```python
from build123d import *

# Parameters (mm, degrees)
F0_R     = 53.6575
F1_DEPTH = 127
F2_R     = 48.26
F3_DEPTH = 118.11
F4_R     = 5.08
F5_R     = 5.08


with BuildPart() as f1:
    # F0 (on Top) → F1 (new body)
    with BuildSketch(Plane.XY):
        Circle(F0_R)
    extrude(amount=F1_DEPTH)

    # F2 (on face) → F3 (cut)
    with BuildSketch(Plane.XY.offset(127)):
        Circle(F2_R)
    extrude(amount=-F3_DEPTH, mode=Mode.SUBTRACT)

    # F4
    f4_edges = [f1.edges().sort_by_distance(p)[0] for p in [
        (-53.6575, 0, 127),
    ]]
    fillet(f4_edges, radius=F4_R)

    # F5
    f5_edges = [f1.edges().sort_by_distance(p)[0] for p in [
        (-53.6575, 0, 0),
    ]]
    fillet(f5_edges, radius=F5_R)


solid = f1.part
```
The listing builds one solid part. Answer for the finished solid, in the listing's coordinates (mm). Give positions to 0.01 mm unless a question says otherwise; leave off trailing zeros. Order: outer loops, then holes, each group sorted by start corner. A loop starts at its lowest first (then second) coordinate and runs counter-clockwise, first axis right, second up. Notation, with made-up numbers: (-38, -35) - (1, -35) arc R20 cw to (1, -14) - close; hole circle Ø2 at (70.25, 46.5). An arc over 180 degrees is marked (long way). Answer in a Markdown table with one row per item. Add a question column.
Q1. Given P1, Ø1, axis at x = -1, y = 29.5, coming from the +Z side; P2, Ø12, axis at x = -38.5, y = 40.5, coming from the -Z side; P3, Ø1.5, axis at x = -13.5, z = 92.5, coming from the -Y side, each flat-ended and moving along its own axis, determine where each tip first touches the part or whether it passes through.
Q2. For a pull along Z with two mould halves and no side action, classify faces 1 (the flat face through (-1, 1, 8.89)), 2 (the flat face through (-1, 1, 0)), 3 (the cylindrical face through (46.03, 14.5, 68.77)) as released by +Z, released by -Z, zero draft, split by the parting line, or undercut.
Q3. Find the intervals of material crossed by line 1 along Y through (x, z) = (0, 77.5); line 2 along Z through (x, y) = (-3, 45); line 3 along X through (y, z) = (42.5, 77.5), in increasing order. Write a range as [from, to].
Q4. The part is cut by section C-C (z = 16.5). Determine the outline of the cut face in (x, y) (1 decimal), then the cut area to 3 significant figures.
Q5. The part is cut by section A-A (x = 0). Determine the outline of the cut face in (y, z), then the cut area to 3 significant figures.
Determined:
| question | item | result |
|---|---|---|
| 1 | P1 | stops at z = 8.89 |
| 1 | P2 | stops at z = 0.17 |
| 1 | P3 | stops at y = -52.12 |
| 2 | face 1 | released by +Z |
| 2 | face 2 | released by -Z |
| 2 | face 3 | zero draft |
| 3 | line 1 | y = [-53.66, -48.26], [48.26, 53.66] |
| 3 | line 2 | z = [0, 8.89] |
| 3 | line 3 | x = [-32.75, -22.86], [22.86, 32.75] |
| 4 | outline | circle Ø107.3 at (0, 0); hole circle Ø96.5 at (0, 0) |
| 4 | area | 1,730 mm² |
| 5 | outline | (-53.66, 5.08) arc R5.08 ccw to (-48.58, 0) - (48.58, 0) arc R5.08 ccw to (53.66, 5.08) - (53.66, 121.92) arc R5.08 ccw to (48.58, 127) - (48.26, 127) - (48.26, 8.89) - (-48.26, 8.89) - (-48.26, 127) - (-48.58, 127) arc R5.08 ccw to (-53.66, 121.92) - close |
| 5 | area | 2,210 mm² |
